from build123d import *

# Parameters (mm, degrees)
F0_W     = 43.18
F0_H     = 73.66
F0_R     = 1.905
F1_DEPTH = 3.81
F2_SIZE  = 1.27
F3_SIZE  = 2.54


with BuildPart() as f1:
    # F0 (on Top) → F1 (new body)
    with BuildSketch(Plane.XY):
        with Locations((-58.500675, 50.269581)):
            Rectangle(F0_W, F0_H)
        with Locations((-76.280675, 17.249581)):
            Circle(F0_R, mode=Mode.SUBTRACT)
        with Locations((-39.450675, 17.249581)):
            Circle(F0_R, mode=Mode.SUBTRACT)
        with Locations((-76.280675, 83.289581)):
            Circle(F0_R, mode=Mode.SUBTRACT)
        with Locations((-39.450675, 83.289581)):
            Circle(F0_R, mode=Mode.SUBTRACT)
    extrude(amount=F1_DEPTH)

    # F2
    f2_edges = [f1.edges().sort_by_distance(p)[0] for p in [
        (-36.910675, 13.439581, 1.905),
        (-36.910675, 87.099581, 1.905),
    ]]
    chamfer(f2_edges, length=F2_SIZE)

    # F3
    f3_edges = [f1.edges().sort_by_distance(p)[0] for p in [
        (-80.090675, 13.439581, 1.905),
        (-80.090675, 87.099581, 1.905),
    ]]
    chamfer(f3_edges, length=F3_SIZE)


solid = f1.part
Here's how the part is built. I have some questions about the finished solid (model axes, mm). Coordinates: 2 decimals unless noted, no trailing zeros. Loops run counter-clockwise (first coordinate to the right, second up) from the corner with the lowest first, then second, coordinate; pieces in that order, holes last.
1. I need wall thicknesses on L1, parallel to X at y = 17.5, z = 2.65; L2, parallel to Y at x = -41, z = 0.85; L3, parallel to X at y = 18, z = 2.6. Which ranges of each line are inside material? Lowest first, please.
2. For P1, Ø2.5, axis at x = -39.45, y = 83.29, coming from the -Z side, with a flat end and sliding along its axis, tell me the tip position at first contact or that it passes through.
3. Imagine slicing it at A-A, the plane z = 2.3. Please give me the cut outline in (x, y) (3 decimals), and give its area (3 significant figures).
4. If we mould it in two halves opening along X, with no side actions, what happens to faces 1 (the flat face through (-59, 51, 3.81)), 2 (the cylindrical face through (-37.634, 17.822, 1.878)), 3 (the flat face through (-80.091, 50, 2)), 4 (the cylindrical face through (-75.26, 84.9, 1.88))? For each: pulls with the +X half, pulls with the -X half, needs draft (parallel to the pull), parting line crosses it, or undercut.
Taken from the geometry:
1. L1: x = -80.09 to -78.17, -74.39 to -41.34, -37.56 to -36.91
1. L2: y = 13.44 to 16.14, 18.36 to 82.18, 84.4 to 87.1
1. L3: x = -80.09 to -78.03, -74.53 to -41.2, -37.7 to -36.91
2. P1: passes through
3. outline: (-80.091, 15.98) - (-77.551, 13.44) - (-38.181, 13.44) - (-36.911, 14.71) - (-36.911, 85.83) - (-38.181, 87.1) - (-77.551, 87.1) - (-80.091, 84.56) - close; hole circle Ø3.81 at (-76.281, 17.25); hole circle Ø3.81 at (-76.281, 83.29); hole circle Ø3.81 at (-39.451, 17.25); hole circle Ø3.81 at (-39.451, 83.29)
3. area: 3,130 mm2
4. face 1: needs draft
4. face 2: undercut
4. face 3: pulls with the -X half
4. face 4: undercut
